Verification items for the finished model (mm, model axes). Face numbers are marked on the shaded views. A direction names the side the tool comes from. Give positions to 0.01 mm unless a question says otherwise; leave off trailing zeros. Write each loop counter-clockwise with the first axis right and the second up, starting at its lowest first coordinate (ties: lowest second). Pieces come first, ordered by that corner, then holes. Notation, with made-up numbers: (46.5, 78.5) - (54.5, 78.5) arc R27 cw to (54.5, 112.5) - close; hole circle Ø2 at (13, 28). An arc over 180 degrees is marked (long way). Put each result on its own line as item: value.
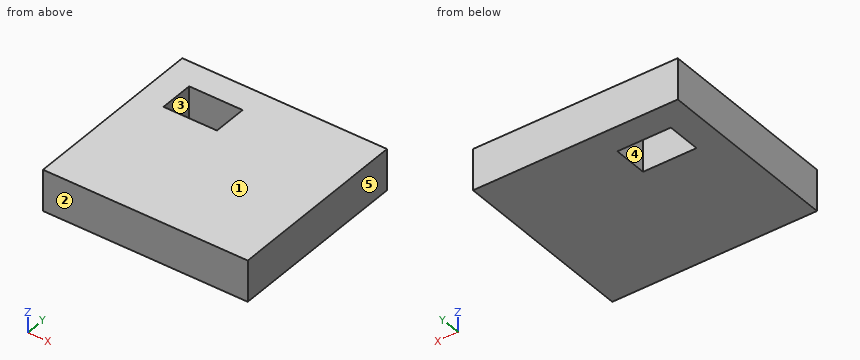
from build123d import *

# Parameters (mm, degrees)
F1_W     = 73.41028
F1_H     = 38.70118
F2_DEPTH = 25.4
F0_W     = 126.091852
F0_H     = 115.206472
F3_DEPTH = 25.4
F4_W     = 32.916133
F4_H     = 21.217024
F5_DEPTH = 25.4


with BuildPart() as f2:
    # F1 (on Top) → F2 (new body)
    with BuildSketch(Plane.XY):
        Rectangle(F1_W, F1_H)
    extrude(amount=F2_DEPTH)

    # F0 (on Top) → F3 (join)
    with BuildSketch(Plane.XY):
        Rectangle(F0_W, F0_H)
    extrude(amount=F3_DEPTH)

    # F4 (on Top) → F5 (cut)
    with BuildSketch(Plane.XY):
        with Locations((-29.931498, 30.338363)):
            Rectangle(F4_W, F4_H)
    extrude(amount=F5_DEPTH, mode=Mode.SUBTRACT)


solid = f2.part
Q1. Section check C-C, the plane z = 2. Record the cut outline in (x, y).
Answers follow:
outline: (-63.05, -57.6) - (63.05, -57.6) - (63.05, 57.6) - (-63.05, 57.6) - close; hole (-46.39, 19.73) - (-13.47, 19.73) - (-13.47, 40.95) - (-46.39, 40.95) - close
Q2. Section check A-A, the plane y = 37. Record the cut outline in (x, z), plus the area to 3 significant figures.
Answers follow:
outline: (-63.05, 0) - (-46.39, 0) - (-46.39, 25.4) - (-63.05, 25.4) - close; (-13.47, 0) - (63.05, 0) - (63.05, 25.4) - (-13.47, 25.4) - close
area: 2,370 mm2
Q3. Set-up check for the marked faces 4 and 5: record each of +Z, -Z, +X, -X, +Y, -Y from which the full face is reachable in a straight line by a thin tool's end or side.
Answers follow:
face 4: +Z, -Z
face 5: +Z, -Z, +X, +Y, -Y
Q4. Section check B-B, the plane x = -20.5. Record the cut outline in (y, z), plus the area to 3 significant figures.
Answers follow:
outline: (-57.6, 0) - (19.73, 0) - (19.73, 25.4) - (-57.6, 25.4) - close; (40.95, 0) - (57.6, 0) - (57.6, 25.4) - (40.95, 25.4) - close
area: 2,390 mm2
Q5. Go/stop test with a flat-tipped pin: pin 1 Ø5 at (x, y) = (-20.5, 39) entering from -Z. Record where the tip stops, or that it passes through.
Answers follow:
pin 1: stops at z = 0
Q6. Scan lines: line 1 along Y through (x, z) = (-44.5, 21.5); line 2 along X through (y, z) = (24, 3.5). Record each from-to range of solid material in increasing order.
Answers follow:
line 1: y = -57.6 to 19.73, 40.95 to 57.6
line 2: x = -63.05 to -46.39, -13.47 to 63.05
Q7. Release check for a two-part mould opening along Y. For the marked faces 1, 2 and 3 record: released by +Y, released by -Y, zero draft, split by the parting line, or undercut.
Answers follow:
face 1: zero draft
face 2: released by -Y
face 3: undercut
